```python
from build123d import *

# Parameters (mm, degrees)
SKETCH2_W                           = 20
SKETCH2_H                           = 9.5
BOSS_EXTRUDE5_DEPTH                 = 10
SKETCH2_8_W                         = 60
SKETCH2_8_H                         = 6
BOSS_EXTRUDE6_DEPTH                 = 8
F_8_0MM_CLEARANCE_DOWEL_HOLE1_D     = 8
F_8_0MM_CLEARANCE_DOWEL_HOLE1_DEPTH = 3.2
F_8_0MM_CLEARANCE_DOWEL_HOLE1_TIP   = 2.403442476
F_8_0MM_CLEARANCE_DOWEL_HOLE2_D     = 8
F_8_0MM_CLEARANCE_DOWEL_HOLE2_DEPTH = 3
F_8_0MM_CLEARANCE_DOWEL_HOLE2_TIP   = 2.403442476
F_5_0MM_CLEARANCE_DOWEL_HOLE5_D     = 5
M4_TAPPED_HOLE1_D                   = 3.3
M4_TAPPED_HOLE1_DEPTH               = 10.1
M4_TAPPED_HOLE1_TIP                 = 0.991420021
M4_TAPPED_HOLE2_D                   = 3.3
M4_TAPPED_HOLE2_DEPTH               = 10.1
M4_TAPPED_HOLE2_TIP                 = 0.991420021


with BuildPart() as part:
    # Sketch2 → Boss-Extrude5 (new body)
    with BuildSketch(Plane(origin=(0, 0, 0), x_dir=(1, 0, 0), z_dir=(0, 1, 0))):
        with Locations((10, 4.75)):
            Rectangle(SKETCH2_W, SKETCH2_H)
        Polygon((40, 30.5), (-20, 30.5), (-20, 9.5), (0, 9.5), (20, 9.5), (40, 9.5), align=None)
    extrude(amount=BOSS_EXTRUDE5_DEPTH)

    # Sketch2_8 → Boss-Extrude6 (add)
    with BuildSketch(Plane(origin=(0, 0, 0), x_dir=(1, 0, 0), z_dir=(0, 1, 0))):
        with Locations((10, 33.5)):
            Rectangle(SKETCH2_8_W, SKETCH2_8_H)
    extrude(amount=BOSS_EXTRUDE6_DEPTH)

    # 8.0mm Clearance Dowel Hole1
    with Locations(Plane(origin=(0, 10, 0), x_dir=(1, 0, 0), z_dir=(0, 1, 0))):
        with Locations((10, 24)):
            Hole(F_8_0MM_CLEARANCE_DOWEL_HOLE1_D / 2, depth=F_8_0MM_CLEARANCE_DOWEL_HOLE1_DEPTH)
            with Locations((0, 0, -(F_8_0MM_CLEARANCE_DOWEL_HOLE1_DEPTH + F_8_0MM_CLEARANCE_DOWEL_HOLE1_TIP / 2))):  # 118° drill point
                Cone(0, F_8_0MM_CLEARANCE_DOWEL_HOLE1_D / 2, F_8_0MM_CLEARANCE_DOWEL_HOLE1_TIP, mode=Mode.SUBTRACT)

    # 8.0mm Clearance Dowel Hole2
    with Locations(Plane(origin=(0, 0, 0), x_dir=(-1, 0, 0), z_dir=(0, -1, 0))):
        with Locations((-10, 24)):
            Hole(F_8_0MM_CLEARANCE_DOWEL_HOLE2_D / 2, depth=F_8_0MM_CLEARANCE_DOWEL_HOLE2_DEPTH)
            with Locations((0, 0, -(F_8_0MM_CLEARANCE_DOWEL_HOLE2_DEPTH + F_8_0MM_CLEARANCE_DOWEL_HOLE2_TIP / 2))):  # 118° drill point
                Cone(0, F_8_0MM_CLEARANCE_DOWEL_HOLE2_D / 2, F_8_0MM_CLEARANCE_DOWEL_HOLE2_TIP, mode=Mode.SUBTRACT)

    # 5.0mm Clearance Dowel Hole5 (through all)
    with Locations(Plane(origin=(0, 0, 0), x_dir=(-1, 0, 0), z_dir=(0, -1, 0))):
        with Locations((-10, 24)):
            Hole(F_5_0MM_CLEARANCE_DOWEL_HOLE5_D / 2)

    # M4 Tapped Hole1
    with Locations(Plane.XY):
        with Locations((4, 4.604977991)):
            Hole(M4_TAPPED_HOLE1_D / 2, depth=M4_TAPPED_HOLE1_DEPTH)
            with Locations((0, 0, -(M4_TAPPED_HOLE1_DEPTH + M4_TAPPED_HOLE1_TIP / 2))):  # 118° drill point
                Cone(0, M4_TAPPED_HOLE1_D / 2, M4_TAPPED_HOLE1_TIP, mode=Mode.SUBTRACT)

    # M4 Tapped Hole2
    with Locations(Plane.XY):
        with Locations((16, 5.006947279)):
            Hole(M4_TAPPED_HOLE2_D / 2, depth=M4_TAPPED_HOLE2_DEPTH)
            with Locations((0, 0, -(M4_TAPPED_HOLE2_DEPTH + M4_TAPPED_HOLE2_TIP / 2))):  # 118° drill point
                Cone(0, M4_TAPPED_HOLE2_D / 2, M4_TAPPED_HOLE2_TIP, mode=Mode.SUBTRACT)


solid = part.part
```
For this review, take the finished solid that the model builds, in its own axes (mm). A direction names the side the tool comes from. Round coordinates to 2 decimals unless told otherwise and drop trailing zeros. Write each loop counter-clockwise with the first axis right and the second up, starting at its lowest first coordinate (ties: lowest second). Pieces come first, ordered by that corner, then holes. Notation, with made-up numbers: (-31, 76.5) -> (13, 76.5) arc R20 cw to (13, 98.5) -> close; hole circle Ø2 at (8.25, 32). An arc over 180 degrees is marked (long way). One line per question, with ' | ' between items. Start each with the question number.
1) Add section C-C (x = 10). Write out the cut boundary in (y, z).
2) Mouldability with a two-part tool opening along X and no side actions: class faces 1 (the flat face through (-10, 5, -9.5)), 2 (the conical face through (15.79, 5.2, -10.92)), 3 (the flat face through (-20, 5, -23)), 4 (the cylindrical face through (9.67, 4.91, -26.48)) as +X half, -X half, draft (parallel to the pull), parting line (faces both ways), or undercut.
3) Wall thickness on line 1 along Z through (x, y) = (10, 8.85); line 2 along X through (y, z) = (4.8, -24); line 3 along Y through (x, z) = (16, -4): over which ranges is each line inside the solid? List them lowest first.
4) Add section D-D (x = -4). Write out the cut boundary in (y, z).
5) Machinability: for faces 5 (the flat face through (0, 5, -5)), 6 (the flat face through (20, 5, -5)), 7 (the cylindrical face through (10.521, 8.378, -27.966)), 8 (the cylindrical face through (7.05, 1.52, -26.7)), 9 (the cylindrical face through (5.31, 3.6, -5.12)), which of the approach directions +Z, -Z, +X, -X, +Y, -Y give a long, thin tool a straight path to every point of the face, cutting with its end or side? Answer none if there is none.
6) Add section A-A (z = -24). Write out the cut boundary in (x, y), and give its area (3 significant figures).
7) For pin 1 Ø3 at (y, z) = (7.5, -3) entering from -X; pin 2 Ø3 at (x, y) = (-7.5, 5) entering from +Z; pin 3 Ø1.6 at (x, y) = (24.5, 9.5) entering from -Z, all flat-tipped, find the tip position at first contact; note any pin that passes through.
8) Add section B-B (y = 1.5). Write out the cut boundary in (x, z).
Reported:
1) outline: (0, -36.5) -> (8, -36.5) -> (8, -30.5) -> (10, -30.5) -> (10, -28) -> (6.8, -28) -> (5.9, -26.5) -> (3.9, -26.5) -> (3, -28) -> (0, -28) -> close; (0, -20) -> (3, -20) -> (3.9, -21.5) -> (5.9, -21.5) -> (6.8, -20) -> (10, -20) -> (10, 0) -> (0, 0) -> close
2) face 1: draft | face 2: undercut | face 3: -X half | face 4: undercut
3) line 1: z = -30.5 to -28, -20 to 0 | line 2: x = -20 to 7.5, 12.5 to 40 | line 3: y = 0 to 3.36, 6.66 to 10
4) outline: (0, -36.5) -> (8, -36.5) -> (8, -30.5) -> (10, -30.5) -> (10, -9.5) -> (0, -9.5) -> close
5) face 5: +Z, -X, +Y, -Y | face 6: +Z, +X, +Y, -Y | face 7: +Y | face 8: -Y | face 9: +Z
6) outline: (-20, 0) -> (6, 0) -> (6, 3) -> (7.5, 3.9) -> (7.5, 5.9) -> (6, 6.8) -> (6, 10) -> (-20, 10) -> close; (12.5, 3.9) -> (14, 3) -> (14, 0) -> (40, 0) -> (40, 10) -> (14, 10) -> (14, 6.8) -> (12.5, 5.9) -> close | area: 529 mm²
7) pin 1: stops at x = 0 | pin 2: stops at z = -9.5 | pin 3: stops at z = -30.5
8) outline: (-20, -36.5) -> (40, -36.5) -> (40, -9.5) -> (20, -9.5) -> (20, 0) -> (0, 0) -> (0, -9.5) -> (-20, -9.5) -> close; hole circle Ø8 at (10, -24)
